```python
from build123d import *

# Parameters (mm, degrees)
F1_DEPTH = 5


with BuildPart() as f1:
    # F0 (on Front) → F1 (new body)
    with BuildSketch(Plane.XZ):
        with BuildLine():
            Line((0, 80), (0, 0))
            Line((0, 0), (22, 0))
            ThreePointArc((22, 0), (80, 58), (138, 0))
            Line((138, 0), (232, 0))
            ThreePointArc((232, 0), (290, 58), (348, 0))
            Line((348, 0), (450, 0))
            Line((450, 0), (450, 80))
            Line((450, 80), (0, 80))
        make_face()
    extrude(amount=F1_DEPTH)


solid = f1.part
```
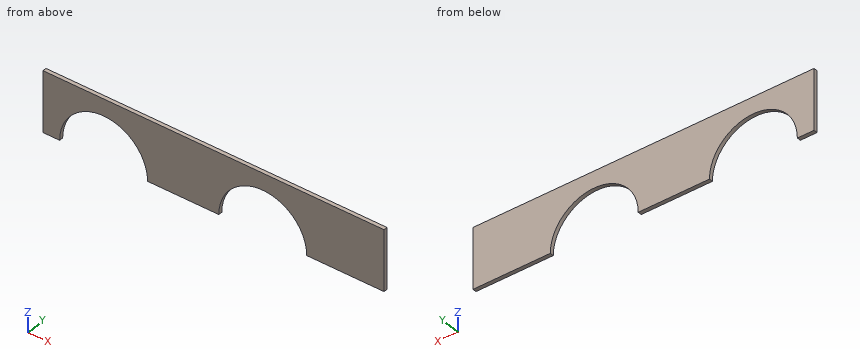
Design review of the part built by this model. Coordinates are the model's own, in mm. Give positions to 0.01 mm unless a question says otherwise; leave off trailing zeros. Order: outer loops, then holes, each group sorted by start corner. A loop starts at its lowest first (then second) coordinate and runs counter-clockwise, first axis right, second up. Notation, with made-up numbers: (17, 18) -> (29, 18) arc R10 ccw to (29, 23) -> close; hole circle Ø11 at (88.25, 0). An arc over 180 degrees is marked (long way). Write item = value, one per line. Start each with the question number.
(1) We need section D-D on z = 50.5. Write out the cut boundary in (x, y).
(2) To check wall thickness, follow line 1 along X through (y, z) = (-4.4, 13.5); line 2 along X through (y, z) = (-1.4, 25); line 3 along Z through (x, y) = (332, -1.95). State the ranges of each line that lie inside material, in increasing order.
(3) We need section C-C on x = 290. Write out the cut boundary in (y, z).
(4) We need section B-B on y = -3.4. Write out the cut boundary in (x, z), plus the area to 3 significant figures.
(5) We need section A-A on z = 8.5. Write out the cut boundary in (x, y), plus the area to 3 significant figures.
Numbers:
q1.outline = (0, -5) -> (51.47, -5) -> (51.47, 0) -> (0, 0) -> close; (108.53, -5) -> (261.47, -5) -> (261.47, 0) -> (108.53, 0) -> close; (318.53, -5) -> (450, -5) -> (450, 0) -> (318.53, 0) -> close
q2.line_1 = 0 to 23.59, 136.41 to 233.59, 346.41 to 450
q2.line_2 = 0 to 27.66, 132.34 to 237.66, 342.34 to 450
q2.line_3 = 40 to 80
q3.outline = (-5, 58) -> (0, 58) -> (0, 80) -> (-5, 80) -> close
q4.outline = (0, 0) -> (22, 0) arc R58 cw to (138, 0) -> (232, 0) arc R58 cw to (348, 0) -> (450, 0) -> (450, 80) -> (0, 80) -> close
q4.area = 25,400 mm^2
q5.outline = (0, -5) -> (22.63, -5) -> (22.63, 0) -> (0, 0) -> close; (137.37, -5) -> (232.63, -5) -> (232.63, 0) -> (137.37, 0) -> close; (347.37, -5) -> (450, -5) -> (450, 0) -> (347.37, 0) -> close
q5.area = 1,100 mm^2
